Verification items for this drawing (mm, ordinates from the low corner). Round coordinates to 2 decimals unless told otherwise and drop trailing zeros. Loops run counter-clockwise (first coordinate to the right, second up) from the corner with the lowest first, then second, coordinate; pieces in that order, holes last. Notation, with made-up numbers: M 5,71 L 9,71 A26 cw 9,99 Z; hole C -18,-5 d5. An arc over 180 degrees is marked long. Answer as CSV lines item,"result".
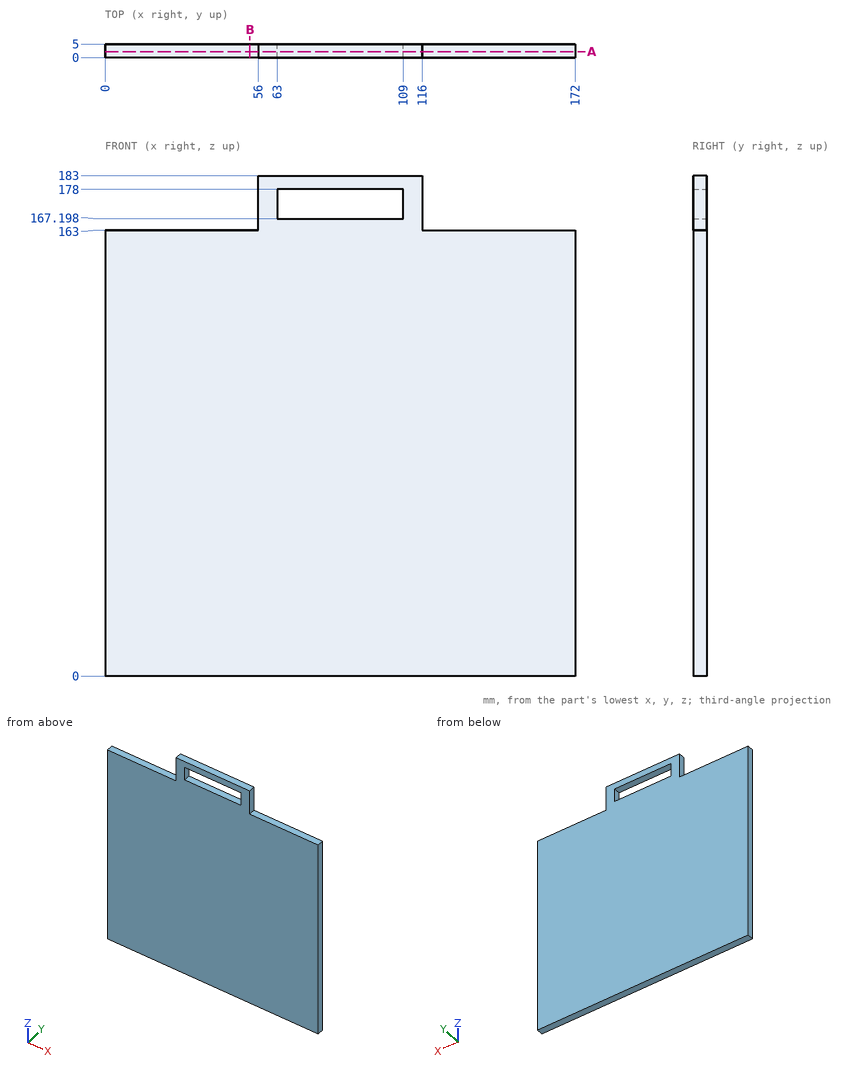
1) Section check A-A (y = 2.2). Record the cut outline in (x, z), plus the area to 3 significant figures.
Here are the results:
outline,"M 0,0 L 172,0 L 172,163 L 116,163 L 116,183 L 56,183 L 56,163 L 0,163 Z; hole M 63,167.2 L 109,167.2 L 109,178 L 63,178 Z"
area,"28,700 mm^2"
2) Go/stop test with flat-tipped pins: pin 1 (1.5 mm diameter, centred on x = 54, y = 1, fed in from +Z); pin 2 (1.5 mm diameter, centred on y = 2, z = 173.5, fed in from -X); pin 3 (2.5 mm diameter, centred on y = 2, z = 172.5, fed in from +X). Record where each tip stops, or that it passes through.
Here are the results:
pin 1,"stops at z = 163"
pin 2,"stops at x = 56"
pin 3,"stops at x = 116"
3) Material ranges on probe 1 along Z at (x, y) = (107, 2.6); probe 2 along X at (y, z) = (4.3, 173.5); probe 3 along Z at (x, y) = (15.5, 3.9), recorded low to high.
Here are the results:
probe 1,"z = 0 to 167.2, 178 to 183"
probe 2,"x = 56 to 63, 109 to 116"
probe 3,"z = 0 to 163"
4) Section check B-B (x = 53). Record the cut outline in (y, z), plus the area to 3 significant figures.
Here are the results:
outline,"M 0,0 L 5,0 L 5,163 L 0,163 Z"
area,"815 mm^2"
